```python
from build123d import *

# Parameters (mm, degrees)
SKETCH_1_R          = 6.1
EXTRUDE_1_DEPTH     = 10
SKETCH_2_R          = 3
CUT_EXTRUDE_2_DEPTH = 116.089044031
CHAMFER_1_SIZE      = 2.5
CUT_EXTRUDE_3_DEPTH = 131.445982376


with BuildPart() as part:
    # 草圖1 → 填料-伸長1 (new body)
    with BuildSketch(Plane.XY):
        Polygon((-29.956118011, 9.755168573), (-48.742646001, 2.894675435), (-26.446043305, -58.161540532), (-82.490240349, -78.627846462), (-73.914623927, -102.111006449), (0.916101107, -74.784207382), align=None)
        with Locations((-35.919135437, -3.068341991)):
            Circle(SKETCH_1_R, mode=Mode.SUBTRACT)
    extrude(amount=EXTRUDE_1_DEPTH)

    # 草圖2 → 除料-伸長2 (cut, through all)
    with BuildSketch(Plane(origin=(15.628555148, -42.796674065, 0), x_dir=(0.9393263994919209, 0.3430246568652819, 0), z_dir=(-0.3430246568652819, 0.939326399491921, 0))):
        with Locations(Location((-95.671540667, -4.982155923, 0), (0, 0, 180))):
            Circle(SKETCH_2_R)
        with Locations(Location((-52.126292594, -4.982155923, 0), (0, 0, 180))):
            Circle(SKETCH_2_R)
    extrude(amount=-CUT_EXTRUDE_2_DEPTH, mode=Mode.SUBTRACT)

    # 導角1
    chamfer_1_edges = [part.edges().sort_by_distance(p)[0] for p in [
        (0.916101107, -74.784207382, 5),
        (-73.914623927, -102.111006449, 5),
        (-82.490240349, -78.627846462, 5),
        (-48.742646001, 2.894675435, 5),
        (-29.956118011, 9.755168573, 5),
    ]]
    chamfer(chamfer_1_edges, length=CHAMFER_1_SIZE)

    # 草圖3 → 除料-伸長3 (cut, through all)
    with BuildSketch(Plane(origin=(0, 0, 0), x_dir=(-1, 0, 0), z_dir=(0, 0, -1))):
        Polygon((52.754237092, -69.656073014), (54.393890854, -79.013505116), (47.10994382, -85.112202978), (38.186343025, -81.853468738), (36.546689263, -72.496036636), (43.830636297, -66.397338774), align=None)
    extrude(amount=-CUT_EXTRUDE_3_DEPTH, mode=Mode.SUBTRACT)


solid = part.part
```
Input: part model. Units: mm. Frame: model coordinates. A direction names the side the tool comes from. Coordinates: 2 decimals unless noted, no trailing zeros. Write each loop counter-clockwise with the first axis right and the second up, starting at its lowest first coordinate (ties: lowest second). Pieces come first, ordered by that corner, then holes. Notation, with made-up numbers: (64, -20) -> (108, -20) arc R8 ccw to (108, -8) -> close; hole circle Ø2 at (54.25, 11.25). An arc over 180 degrees is marked (long way). Write each question's results on one line, items separated by ' | '.
Item 1: Section query B-B on x = -6.5. Return loops of the section in (y, z), plus the area to 3 significant figures.
Conclusion:
outline: (-77.49, 0) -> (-54.48, 0) -> (-54.48, 10) -> (-77.49, 10) -> close | area: 230 mm^2
Item 2: Section query C-C on y = -48.5. Return loops of the section in (x, z), plus the area to 3 significant figures.
Conclusion:
outline: (-29.97, 0) -> (-8.68, 0) -> (-8.68, 10) -> (-29.97, 10) -> close | area: 213 mm^2
Item 3: Section query A-A on y = -6. Return loops of the section in (x, z).
Conclusion:
outline: (-45.49, 0) -> (-41.27, 0) -> (-41.27, 10) -> (-45.49, 10) -> close; (-30.57, 0) -> (-24.2, 0) -> (-24.2, 10) -> (-30.57, 10) -> close
Item 4: Material intervals for probe 1 along Z at (x, y) = (-69, -96); probe 2 along X at (y, z) = (0.5, 7.5); probe 3 along Z at (x, y) = (-72, -79), sorted ascending.
Conclusion:
probe 1: z = 0 to 2.81, 7.15 to 10 | probe 2: x = -47.87 to -40.87, -30.97 to -26.58 | probe 3: z = 0 to 2.13, 7.83 to 10
Item 5: Set-up query: faces 1 (the flat face through (-80.9, -79.4, 4.9)), 2 (the flat face through (-53.563, -74.269, 4.93)), 3 (the flat face through (-37.316, -28.397, 4.93)). Return all of +Z, -Z, +X, -X, +Y, -Y with unobstructed straight access to the full face (end or side cutting, diameter ignored); none if empty.
Conclusion:
face 1: +Z, -Z, -X, +Y | face 2: +Z, -Z | face 3: +Z, -Z, -X
Item 6: Mould query, pull axis Z, two halves, no side actions, for faces 4 (the flat face through (-40.14, -69.49, 4.93)), 5 (the cylindrical face through (-31.795, -73.236, 5.883)), 6 (the cylindrical face through (-71.53, -87.74, 7.51)), 7 (the flat face through (-29, -50, 0)). Classes: +Z half, -Z half, draft (parallel to the pull), parting line (faces both ways), or undercut.
Conclusion:
face 4: draft | face 5: undercut | face 6: undercut | face 7: -Z half
Item 7: Pin query (flat end, axial travel): pin 1 Ø6 at (y, z) = (-42.5, 3.5) entering from -X; pin 2 Ø1.5 at (x, z) = (-16.5, 8) entering from -Y; pin 3 Ø3 at (y, z) = (-16, 2) entering from -X. Return the tip coordinate at first contact, or that it passes through.
Conclusion:
pin 1: stops at x = -33.26 | pin 2: stops at y = -81.42 | pin 3: stops at x = -42.39
